The listing builds one solid part. Answer for the finished solid, in the listing's coordinates (mm). Face numbers are marked on the shaded views. A direction names the side the tool comes from. Give positions to 0.01 mm unless a question says otherwise; leave off trailing zeros. Write each loop counter-clockwise with the first axis right and the second up, starting at its lowest first coordinate (ties: lowest second). Pieces come first, ordered by that corner, then holes. Notation, with made-up numbers: (56, 6.5) -> (105, 6.5) arc R8 ccw to (105, 19.5) -> close; hole circle Ø10 at (8.25, 89). An arc over 180 degrees is marked (long way). Use CSV: the item, a comma, the result in double quotes. Start each with the question number.
from build123d import *

# Parameters (mm, degrees)
SKETCH6_W               = 40
SKETCH6_H               = 2
BOSS_EXTRUDE4_DEPTH     = 16
SKETCH8_R               = 2.6
BOSS_EXTRUDE5_DEPTH     = 2
FILLET1_R               = 1
CUT_EXTRUDE1_DEPTH      = 26.690465157
CUT_EXTRUDE1_DEPTH_BACK = 16
SKETCH7_W               = 42.708590122
SKETCH7_H               = 18.182038554
SKETCH14_R              = 1.749999912
SKETCH14_R_2            = 1.749999996
SKETCH14_R_3            = 1.749999993
BOSS_EXTRUDE8_DEPTH     = 2
SKETCH15_W              = 2
SKETCH15_H              = 18
EXTRUDE_THIN1_DEPTH     = 2


with BuildPart() as part:
    # Sketch6 → Boss-Extrude4 (new body)
    with BuildSketch(Plane(origin=(0, 0, 0), x_dir=(1, 0, 0), z_dir=(0, 1, 0))):
        with Locations((0, -10)):
            Rectangle(SKETCH6_W, SKETCH6_H)
    extrude(amount=BOSS_EXTRUDE4_DEPTH)

    # Sketch8 → Boss-Extrude5 (add)
    with BuildSketch(Plane.XY.offset(11)):
        with Locations(Location((-12, 8, 0), (0, 0, 180))):
            Circle(SKETCH8_R)
    extrude(amount=BOSS_EXTRUDE5_DEPTH)

    # Fillet1
    fillet1_edges = [part.edges().sort_by_distance(p)[0] for p in [
        (-9.4, 8, 11),
    ]]
    fillet(fillet1_edges, radius=FILLET1_R)

    # Sketch7 → Cut-Extrude1 (cut, two sides: drawn at the far end of the back side and taken through both)
    with BuildSketch(Plane.XY.offset(11).offset(-CUT_EXTRUDE1_DEPTH_BACK)):
        with Locations((0, 8)):
            Rectangle(SKETCH7_W, SKETCH7_H)
        with BuildLine():
            Line((-5.942038411, 16), (-12, 16))
            ThreePointArc((-12, 16), (-19.39103626, 11.061467459), (-17.656854249, 2.343145751))
            Line((-17.656854249, 2.343145751), (-15.313708499, 0))
            Line((-15.313708499, 0), (20, 0))
            Line((20, 0), (20, 1.767244224))
            ThreePointArc((20, 1.767244224), (19.761112544, 2.715127447), (19.101517394, 3.43657326))
            Line((19.101517394, 3.43657326), (5.07313553, 12.69329036))
            ThreePointArc((5.07313553, 12.69329036), (-0.191638738, 15.155492779), (-5.942038411, 16))
        make_face(mode=Mode.SUBTRACT)
    extrude(amount=CUT_EXTRUDE1_DEPTH + CUT_EXTRUDE1_DEPTH_BACK, mode=Mode.SUBTRACT)


with BuildPart() as body_2:
    # Mirror2: mirrored copy
    add(part.part.mirror(Plane.XY))


with BuildPart() as part_1:
    add(part.part)

    add(body_2.part)  # Boss-Extrude8 merges body 2
    # Sketch14 → Boss-Extrude8 (add)
    with BuildSketch(Plane(origin=(0, 0, 0), x_dir=(1, 0, 0), z_dir=(0, 1, 0))):
        Polygon((-15.313708496, -10), (-15.313708496, 10), (20.000000038, 10), (19.999999862, -10), align=None)
        with Locations(Location((12.999999996, -3e-07, 0), (0, 0, 270))):
            Circle(SKETCH14_R, mode=Mode.SUBTRACT)
        with Locations(Location((3, -1.24e-07, 0), (0, 0, 270))):
            Circle(SKETCH14_R_2, mode=Mode.SUBTRACT)
        with Locations(Location((-6.999999997, -1.24e-07, 0), (0, 0, 270))):
            Circle(SKETCH14_R_3, mode=Mode.SUBTRACT)
        with BuildLine():
            Line((16.000000003, 6), (9.925463662, 6))
            ThreePointArc((9.925463662, 6), (7.975463662, 4.05), (6.025463662, 6))
            Line((6.025463662, 6), (-0.049072678, 6))
            ThreePointArc((-0.049072678, 6), (-1.999999996, 4.049072682), (-3.950927314, 6))
            Line((-3.950927314, 6), (-11.313708496, 6))
            Line((-11.313708496, 6), (-11.313708496, 3.801896638))
            ThreePointArc((-11.313708496, 3.801896638), (-6.408964515, 5.719543307), (-1.999999996, 2.839454047))
            ThreePointArc((-1.999999996, 2.839454047), (3.000000101, 5.749999872), (8.000000096, 2.83945387))
            ThreePointArc((8.000000096, 2.83945387), (11.562298515, 5.567361143), (15.999999994, 4.905353815))
            Line((15.999999994, 4.905353815), (16.000000003, 6))
        make_face(mode=Mode.SUBTRACT)
        with BuildLine():
            Line((-11.313708496, -6), (-11.313708496, -3.801896885))
            ThreePointArc((-11.313708496, -3.801896885), (-6.408964515, -5.719543555), (-1.999999996, -2.839454295))
            ThreePointArc((-1.999999996, -2.839454295), (3, -5.75000012), (7.999999996, -2.839454295))
            ThreePointArc((7.999999996, -2.839454295), (11.562298368, -5.567361705), (15.999999907, -4.905354469))
            Line((15.999999907, -4.905354469), (15.999999897, -6))
            Line((15.999999897, -6), (9.949999996, -6))
            ThreePointArc((9.949999996, -6), (7.999999996, -4.05), (6.049999996, -6))
            Line((6.049999996, -6), (-0.049999996, -6))
            ThreePointArc((-0.049999996, -6), (-1.999999996, -4.05), (-3.949999996, -6))
            Line((-3.949999996, -6), (-11.313708496, -6))
        make_face(mode=Mode.SUBTRACT)
        with BuildLine():
            Line((9.425463662, 8), (6.525463662, 8))
            ThreePointArc((6.525463662, 8), (7.975463662, 6.55), (9.425463662, 8))
        make_face(mode=Mode.SUBTRACT)
        with BuildLine():
            Line((-3.449999996, -8), (-0.549999996, -8))
            ThreePointArc((-0.549999996, -8), (-1.999999996, -6.55), (-3.449999996, -8))
        make_face(mode=Mode.SUBTRACT)
        with BuildLine():
            Line((-0.549999996, 8), (-3.449999996, 8))
            ThreePointArc((-3.449999996, 8), (-1.999999996, 6.55), (-0.549999996, 8))
        make_face(mode=Mode.SUBTRACT)
        with BuildLine():
            Line((6.549999996, -8), (9.449999996, -8))
            ThreePointArc((9.449999996, -8), (7.999999996, -6.55), (6.549999996, -8))
        make_face(mode=Mode.SUBTRACT)
    extrude(amount=BOSS_EXTRUDE8_DEPTH)

    # Sketch15 → Extrude-Thin1 (add)
    with BuildSketch(Plane(origin=(0, 2, 0), x_dir=(1, 0, 0), z_dir=(0, 1, 0))):
        with Locations((-12, 0)):
            Rectangle(SKETCH15_W, SKETCH15_H)
    extrude(amount=EXTRUDE_THIN1_DEPTH)


solid = part_1.part
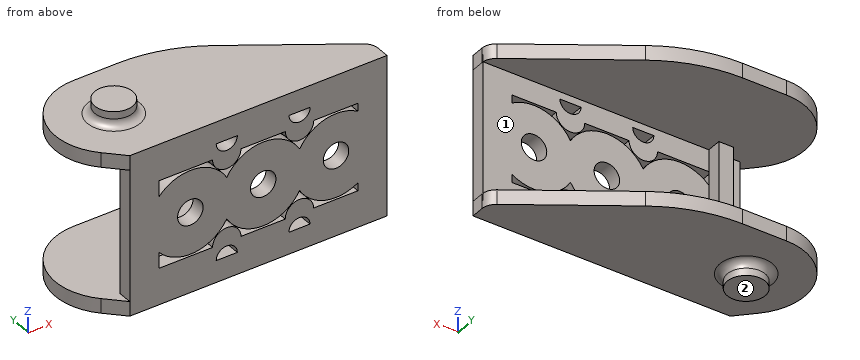
Q1. For the marked faces 1 and 2, determine the directions among +Z, -Z, +X, -X, +Y, -Y from which every point of the face is accessible in a straight line to the end or side of a thin tool.
Q2. Straight lines are drawn through the part: L1, parallel to X at y = 1.35, z = 0; L2, parallel to Z at x = -17, y = 13; L3, parallel to Z at x = 13, y = 0.55. For each, find the intervals that lie inside material, in ascending order.
Q3. Flat-ended cylindrical pins translate along their axes: pin 1 Ø1.5 at (x, z) = (-0.5, -2.5) entering from +Y; pin 2 Ø3 at (y, z) = (5, -1) entering from +X; pin 3 Ø0.5 at (y, z) = (0.5, -5.5) entering from -X; pin 4 Ø3 at (x, z) = (3, 0) entering from +Y. Find the tip coordinate at first contact, or state that the pin passes through.
Q4. Section C-C on y = 8 is taken. Give the vertices of the cut face in (x, z), then the cut area to 3 significant figures.
Q5. Section B-B on x = -1.5 is taken. Give the vertices of the cut face in (y, z), then the cut area to 3 significant figures.
Q6. Section D-D on x = -16.5 is taken. Give the vertices of the cut face in (y, z).
Q7. Section A-A on x = -7 is taken. Give the vertices of the cut face in (y, z).
Output:
1,face 1,"+X, +Y"
1,face 2,"-Z, +X, -X, +Y, -Y"
2,L1,"-15.31 to -8.75, -5.25 to 1.25, 4.75 to 11.25, 14.75 to 20"
2,L2,"-11 to -9, 9 to 11"
2,L3,"-11 to -6, -5.75 to -1.75, 1.75 to 5.75, 6 to 11"
3,pin 1,"y = 2"
3,pin 2,"x = -11"
3,pin 3,"x = -15.31"
3,pin 4,"through"
4,outline,"(-20, -11) -> (-15.6, -11) arc R1 cw to (-14.6, -12) -> (-14.6, -13) -> (-9.4, -13) -> (-9.4, -12) arc R1 cw to (-8.4, -11) -> (12.19, -11) -> (12.19, -9) -> (-20, -9) -> close; (-20, 9) -> (12.19, 9) -> (12.19, 11) -> (-8.4, 11) arc R1 cw to (-9.4, 12) -> (-9.4, 13) -> (-14.6, 13) -> (-14.6, 12) arc R1 cw to (-15.6, 11) -> (-20, 11) -> close"
4,area,"150 mm²"
5,outline,"(0, -11) -> (15.5, -11) -> (15.5, -9) -> (2, -9) -> (2, -8) -> (0, -8) -> close; (0, -6.64) -> (2, -6.64) -> (2, -4.11) -> (0, -4.11) -> close; (0, -3.58) -> (2, -3.58) -> (2, 3.58) -> (0, 3.58) -> close; (0, 4.12) -> (2, 4.12) -> (2, 6.64) -> (0, 6.64) -> close; (0, 8) -> (2, 8) -> (2, 9) -> (15.5, 9) -> (15.5, 11) -> (0, 11) -> close"
5,area,"90.4 mm²"
6,outline,"(1.19, -11) -> (14.61, -11) -> (14.61, -9) -> (1.19, -9) -> close; (1.19, 9) -> (14.61, 9) -> (14.61, 11) -> (1.19, 11) -> close"
7,outline,"(0, -11) -> (16, -11) -> (16, -9) -> (2, -9) -> (2, -6) -> (0, -6) -> close; (0, -5.75) -> (2, -5.75) -> (2, -1.75) -> (0, -1.75) -> close; (0, 1.75) -> (2, 1.75) -> (2, 5.75) -> (0, 5.75) -> close; (0, 6) -> (2, 6) -> (2, 9) -> (16, 9) -> (16, 11) -> (0, 11) -> close"
